Read the model definition and answer for the solid it produces. Units are mm, in the model's axes. Coordinates: 2 decimals unless noted, no trailing zeros. Order: outer loops, then holes, each group sorted by start corner. A loop starts at its lowest first (then second) coordinate and runs counter-clockwise, first axis right, second up.
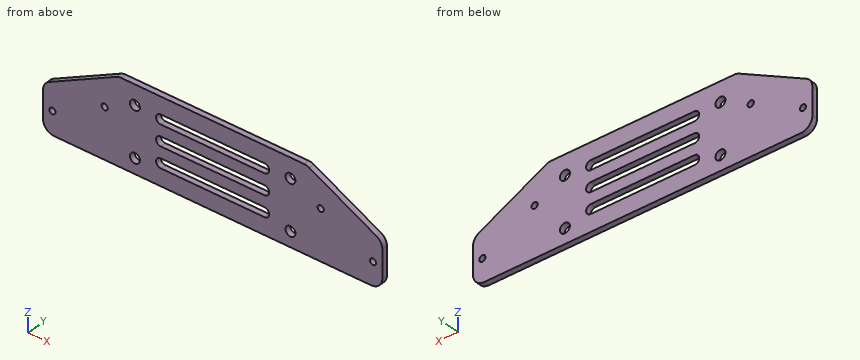
from build123d import *

# Parameters (mm, degrees)
SKETCH_1_W          = 180
SKETCH_1_H          = 45
SKETCH_1_R          = 2.65
EXTRUDE_1_DEPTH     = 3
SKETCH_2_R          = 1.65
CUT_EXTRUDE_1_DEPTH = 3
CUT_EXTRUDE_2_DEPTH = 3
FILLET_1_R          = 6
CUT_EXTRUDE_3_DEPTH = 3


with BuildPart() as part:
    # 草图1 → 凸台-拉伸1 (new body)
    with BuildSketch(Plane(origin=(0, 0, 0), x_dir=(1, 0, 0), z_dir=(0, 1, 0))):
        with Locations((0, -1.25)):
            Rectangle(SKETCH_1_W, SKETCH_1_H)
        with Locations((-41.25, 13.25)):
            Circle(SKETCH_1_R, mode=Mode.SUBTRACT)
        with Locations((41.25, 13.25)):
            Circle(SKETCH_1_R, mode=Mode.SUBTRACT)
        with Locations((-41.25, -13.25)):
            Circle(SKETCH_1_R, mode=Mode.SUBTRACT)
        with Locations((41.25, -13.25)):
            Circle(SKETCH_1_R, mode=Mode.SUBTRACT)
    extrude(amount=EXTRUDE_1_DEPTH)

    # 草图2 → 切除-拉伸1 (cut)
    with BuildSketch(Plane(origin=(0, 3, 0), x_dir=(1, 0, 0), z_dir=(0, 1, 0))):
        with Locations((-85, 9)):
            Circle(SKETCH_2_R)
        with Locations((85, 9)):
            Circle(SKETCH_2_R)
        with Locations((-57.3, -5.3)):
            Circle(SKETCH_2_R)
        with Locations((57.3, -5.3)):
            Circle(SKETCH_2_R)
    extrude(amount=-CUT_EXTRUDE_1_DEPTH, mode=Mode.SUBTRACT)

    # 草图3 → 切除-拉伸2 (cut)
    with BuildSketch(Plane(origin=(0, 3, 0), x_dir=(1, 0, 0), z_dir=(0, 1, 0))):
        Polygon((-90, -3.048881556), (-90, -23.75), (-49.900630707, -23.75), align=None)
        Polygon((90, -23.75), (49.900630707, -23.75), (90, -3.048881556), align=None)
    extrude(amount=-CUT_EXTRUDE_2_DEPTH, mode=Mode.SUBTRACT)

    # 圆角1
    fillet_1_edges = [part.edges().sort_by_distance(p)[0] for p in [
        (-90, 1.5, 3.048881556),
        (-49.900630707, 1.5, 23.75),
        (90, 1.5, 3.048881556),
        (49.900630707, 1.5, 23.75),
        (-90, 1.5, -21.25),
        (90, 1.5, -21.25),
    ]]
    fillet(fillet_1_edges, radius=FILLET_1_R)

    # 草图4 → 切除-拉伸3 (cut)
    with BuildSketch(Plane(origin=(0, 3, 0), x_dir=(1, 0, 0), z_dir=(0, 1, 0))):
        with BuildLine():
            Line((-27.5, 12.25), (27.5, 12.25))
            ThreePointArc((27.5, 12.25), (30, 9.75), (27.5, 7.25))
            Line((27.5, 7.25), (-27.5, 7.25))
            ThreePointArc((-27.5, 7.25), (-30, 9.75), (-27.5, 12.25))
        make_face()
        with BuildLine():
            Line((-27.5, 1.25), (27.5, 1.25))
            ThreePointArc((27.5, 1.25), (30, -1.25), (27.5, -3.75))
            Line((27.5, -3.75), (-27.5, -3.75))
            ThreePointArc((-27.5, -3.75), (-30, -1.25), (-27.5, 1.25))
        make_face()
        with BuildLine():
            Line((-27.5, -9.75), (27.5, -9.75))
            ThreePointArc((27.5, -9.75), (30, -12.25), (27.5, -14.75))
            Line((27.5, -14.75), (-27.5, -14.75))
            ThreePointArc((-27.5, -14.75), (-30, -12.25), (-27.5, -9.75))
        make_face()
    extrude(amount=-CUT_EXTRUDE_3_DEPTH, mode=Mode.SUBTRACT)


solid = part.part
Q1. The part is cut by section C-C, the plane z = 1.25. Determine the outline of the cut face in (x, y).
Q2. The part is cut by section A-A, the plane x = 2.5. Determine the outline of the cut face in (y, z).
Q3. The part is cut by section D-D, the plane x = -61. Determine the outline of the cut face in (y, z).
Q4. Each of these flat-tipped pins is pushed along its axis until it touches: P1, Ø5.5, axis at x = -57.3, z = 5.3, coming from the -Y side; P2, Ø1, axis at y = 1, z = 4.5, coming from the +X side; P3, Ø1, axis at y = 1, z = 3, coming from the +X side. Where does it stop, or does it pass through?
Q5. Straight lines are drawn through the part: L1, parallel to Z at x = 5.5, y = 2.2; L2, parallel to Z at x = -41.25, y = 1.5; L3, parallel to X at y = 0.5, z = -8. For each, find the intervals that lie inside material, in ascending order.
Q6. The part is cut by section B-B, the plane z = -9. Determine the outline of the cut face in (x, y).
Computed values:
1. outline: (-89.71, 0) - (-30, 0) - (-30, 3) - (-89.71, 3) - close; (30, 0) - (89.71, 0) - (89.71, 3) - (30, 3) - close
2. outline: (0, -21.25) - (3, -21.25) - (3, -12.25) - (0, -12.25) - close; (0, -7.25) - (3, -7.25) - (3, -1.25) - (0, -1.25) - close; (0, 3.75) - (3, 3.75) - (3, 9.75) - (0, 9.75) - close; (0, 14.75) - (3, 14.75) - (3, 23.75) - (0, 23.75) - close
3. outline: (0, -21.25) - (3, -21.25) - (3, 18.02) - (0, 18.02) - close
4. P1: stops at y = 0
4. P2: stops at x = 87.85
4. P3: stops at x = 89.13
5. L1: z = -21.25 to -12.25, -7.25 to -1.25, 3.75 to 9.75, 14.75 to 23.75
5. L2: z = -21.25 to -15.9, -10.6 to 10.6, 15.9 to 23.75
5. L3: x = -90 to -86.31, -83.69 to -29.29, 29.29 to 83.69, 86.31 to 90
6. outline: (-90, 0) - (-86.65, 0) - (-86.65, 3) - (-90, 3) - close; (-83.35, 0) - (-29.88, 0) - (-29.88, 3) - (-83.35, 3) - close; (29.88, 0) - (83.35, 0) - (83.35, 3) - (29.88, 3) - close; (86.65, 0) - (90, 0) - (90, 3) - (86.65, 3) - close
